from build123d import *

# Parameters (mm, degrees)
SKETCH1_R           = 25.4
BOSS_EXTRUDE1_DEPTH = 6.35
CUT_EXTRUDE1_DEPTH  = 39.1


with BuildPart() as part:
    # Sketch1 → Boss-Extrude1 (new, symmetric)
    with BuildSketch(Plane.XY):
        Circle(SKETCH1_R)
    extrude(amount=BOSS_EXTRUDE1_DEPTH, both=True)

    # Sketch3 → Cut-Revolve1 (revolve, cut)
    with BuildSketch(Plane(origin=(0, 0, 0), x_dir=(1, 0, 0), z_dir=(0, 1, 0)), mode=Mode.PRIVATE) as cut_revolve1_sk:
        with BuildLine():
            Line((-25.4, 4.445), (-25.4, -4.445))
            Line((-25.4, -4.445), (-22.225, -4.445))
            ThreePointArc((-22.225, -4.445), (-17.78, 0), (-22.225, 4.445))
            Line((-22.225, 4.445), (-25.4, 4.445))
        make_face()
    revolve(cut_revolve1_sk.sketch.rotate(Axis((0, 0, 17.119668281), (0, 0, -1)), 180), axis=Axis((0, 0, 17.119668281), (0, 0, -1)), mode=Mode.SUBTRACT)

    # Sketch4 → Cut-Extrude1 (cut, through all)
    with BuildSketch(Plane(origin=(0, 0, -6.35), x_dir=(-1, 0, 0), z_dir=(0, 0, -1))):
        Polygon((5.645908282, 0), (2.822954141, 4.8895), (-2.822954141, 4.8895), (-5.645908282, 0), (-2.822954141, -4.8895), (2.822954141, -4.8895), align=None)
    extrude(amount=-CUT_EXTRUDE1_DEPTH, mode=Mode.SUBTRACT)


solid = part.part
Design review of the part built by this model. Coordinates are the model's own, in mm. A direction names the side the tool comes from. Coordinates: 2 decimals unless noted, no trailing zeros. Order: outer loops, then holes, each group sorted by start corner. A loop starts at its lowest first (then second) coordinate and runs counter-clockwise, first axis right, second up. Notation, with made-up numbers: (-14, 58) -> (7, 58) arc R19 cw to (7, 63) -> close; hole circle Ø1 at (73.25, 27.5). An arc over 180 degrees is marked (long way). Use one line per item in the form item = value. Start each with the question number.
(1) The part is to be moulded in two halves that separate along Y. For faces 1 (the flat face through (-0.1, 22.5, 4.445)), 2 (the cylindrical face through (-5.506, -24.796, 5.411)), 3 (the flat face through (-4.254, 2.411, -0.089)), say which applies: +Y half, -Y half, draft (parallel to the pull), parting line (faces both ways), or undercut.
(2) Insertion check: pin 1 (3 mm diameter, centred on x = 0, z = -2.5, fed in from +Y); pin 2 (6 mm diameter, centred on x = 1, z = -0.5, fed in from -Y); pin 3 (3 mm diameter, centred on y = -5, z = 2, fed in from +X). Each pin has a flat end and moves straight along its axis. Give the tip position at first contact, or say it passes through.
(3) For probe 1 along Z at (x, y) = (23, 7) (3 decimals); probe 2 along Y at (x, z) = (2, 4.5); probe 3 along Z at (x, y) = (-12.5, 17), list the stretches that pass through material, from the lowest coordinate up.
(4) For faces 4 (the flat face through (0.1, 22.5, -4.445)), 5 (the flat face through (-0.4, -5.3, 6.35)), 6 (the flat face through (4.254, -2.411, -0.089)), list the 3-axis set-ups (+Z, -Z, +X, -X, +Y, -Y) from which the entire face can be reached by the end or side of a thin tool; tool diameter is ignored.
(5) Add section B-B on z = 5.25. State the section outline as (x, y) points, plus the area to 3 significant figures.
Answer block:
q1.face_1 = draft
q1.face_2 = parting line
q1.face_3 = undercut
q2.pin_1 = 20.29
q2.pin_2 = -19.46
q2.pin_3 = 18.87
q3.probe_1 = -6.35 to -4.445, 4.445 to 6.35
q3.probe_2 = -25.32 to -4.89, 4.89 to 25.32
q3.probe_3 = -6.35 to -4.3, 4.3 to 6.35
q4.face_4 = none
q4.face_5 = +Z, +X, -X, +Y, -Y
q4.face_6 = +Z, -Z
q5.outline = circle Ø50.8 at (0, 0); hole (-5.65, 0) -> (-2.82, -4.89) -> (2.82, -4.89) -> (5.65, 0) -> (2.82, 4.89) -> (-2.82, 4.89) -> close
q5.area = 1,940 mm²
